Geometry: final body of the model. Coordinates: model frame, mm. Face numbers are marked on the shaded views. A direction names the side the tool comes from. Round coordinates to 2 decimals unless told otherwise and drop trailing zeros. Write each loop counter-clockwise with the first axis right and the second up, starting at its lowest first coordinate (ties: lowest second). Pieces come first, ordered by that corner, then holes. Notation, with made-up numbers: (79.25, 43.5) - (119.25, 43.5) arc R22 ccw to (119.25, 60.5) - close; hole circle Ø4 at (-5.5, 79.5). An arc over 180 degrees is marked (long way). Use a Markdown table: item, result. Add a question column.
```python
from build123d import *

# Parameters (mm, degrees)
SKETCH8_R           = 2
BOSS_EXTRUDE6_DEPTH = 9
BOSS_EXTRUDE7_START = -9
SKETCH9_R           = 1.395
BOSS_EXTRUDE7_DEPTH = 32
CHAMFER3_SIZE       = 3.5
BOSS_EXTRUDE8_START = -9
SKETCH11_R          = 2
BOSS_EXTRUDE8_DEPTH = 28.5
CUT_EXTRUDE1_START  = -0.2
CUT_EXTRUDE1_DEPTH  = 24.2
FILLET5_R           = 3.2


with BuildPart() as part:
    # Sketch8 → Boss-Extrude6 (new body, symmetric)
    with BuildSketch(Plane.XY):
        with BuildLine():
            Line((-16, -16.195281799), (-16, -22.05))
            Line((-16, -22.05), (16, -22.05))
            ThreePointArc((16, -22.05), (20.242640687, -20.292640687), (22, -16.05))
            Line((22, -16.05), (22, 16.05))
            Line((22, 16.05), (-1.424393869, 2.820825363))
            Line((-1.424393869, 2.820825363), (-1.424393869, -9.35))
            Line((-1.424393869, -9.35), (-1.949620424, -9.35))
            ThreePointArc((-1.949620424, -9.35), (-3.3, -11.095), (-4.650379576, -9.35))
            Line((-4.650379576, -9.35), (-16, -9.35))
            Line((-16, -9.35), (-16, -16.195281799))
        make_face()
        with Locations((16, -16.05)):
            Circle(SKETCH8_R, mode=Mode.SUBTRACT)
    extrude(amount=BOSS_EXTRUDE6_DEPTH, both=True)

    # Sketch9 → Boss-Extrude7 (add)
    with BuildSketch(Plane.XY.offset(BOSS_EXTRUDE7_START)):
        with BuildLine():
            Line((8.5, 4.678478311), (-5.487189769, -7.103420343))
            ThreePointArc((-5.487189769, -7.103420343), (-6.682635801, -9.410517634), (-5.896579657, -11.887189769))
            Line((-5.896579657, -11.887189769), (-0.72278451, -18.029396273))
            Line((-0.72278451, -18.029396273), (8.5, -12.820730998))
            Line((8.5, -12.820730998), (8.5, 4.678478311))
        make_face()
        with Locations((-3.3, -9.7)):
            Circle(SKETCH9_R, mode=Mode.SUBTRACT)
    extrude(amount=BOSS_EXTRUDE7_DEPTH)

    # Chamfer3
    chamfer3_edges = [part.edges().sort_by_distance(p)[0] for p in [
        (8.5, -4.071126344, 23),
    ]]
    chamfer(chamfer3_edges, length=CHAMFER3_SIZE)

    # Sketch11 → Boss-Extrude8 (add)
    with BuildSketch(Plane.XY.offset(BOSS_EXTRUDE8_START)):
        with BuildLine():
            Line((8.5, 8.425731957), (8.5, -22.05))
            Line((8.5, -22.05), (16, -22.05))
            ThreePointArc((16, -22.05), (20.242640687, -20.292640687), (22, -16.05))
            Line((22, -16.05), (22, 16.05))
            Line((22, 16.05), (8.5, 8.425731957))
        make_face()
        with Locations((16, -16.05)):
            Circle(SKETCH11_R, mode=Mode.SUBTRACT)
    extrude(amount=BOSS_EXTRUDE8_DEPTH)

    # Sketch8<4> → Cut-Extrude1 (cut, through all)
    with BuildSketch(Plane.XY.offset(CUT_EXTRUDE1_START)):
        Polygon((-16, -16.195281799), (-16, -22.05), (-14.391687016, -22.05), (-14.391687016, -9.35), (-16, -9.35), align=None)
    extrude(amount=CUT_EXTRUDE1_DEPTH, mode=Mode.SUBTRACT)

    # Fillet5
    fillet5_edges = [part.edges().sort_by_distance(p)[0] for p in [
        (-10.534298793, -9.35, 9),
        (-2.945843508, -22.05, 9),
    ]]
    fillet(fillet5_edges, radius=FILLET5_R)


solid = part.part
```
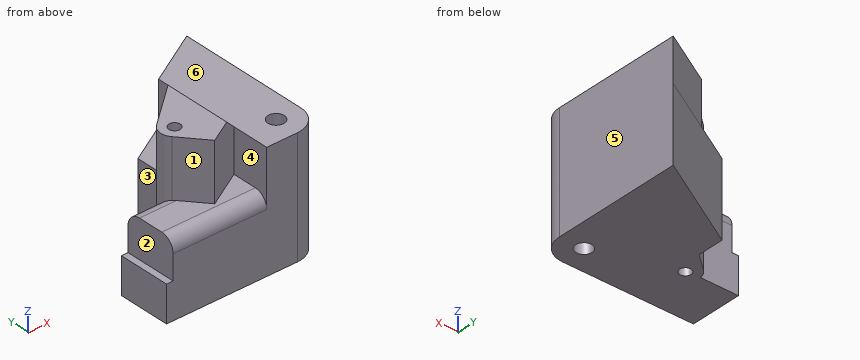
1) Section B-B, the plane z = 8. Return the cut outline in (x, y) (3 decimals), then the cut area to 3 significant figures.
2) Set-up query: the marked faces 1, 2 and 3. Return all of +Z, -Z, +X, -X, +Y, -Y with unobstructed straight access to the full face (end or side cutting, diameter ignored); none if empty.
3) Section D-D, the plane y = 0.5. Return the cut outline in (x, z), then the cut area to 3 significant figures.
4) Section C-C, the plane x = 3. Return the cut outline in (y, z).
5) Pin query (flat end, axial travel): P1, Ø0.8, axis at x = -15, y = -13.5, coming from the +Z side; P2, Ø10.5, axis at x = -12, z = 0.5, coming from the +Y side; P3, Ø1.5, axis at x = -6, z = 14, coming from the -Y side. Return the tip coordinate at first contact, or that it passes through.
6) Draft query along X for the marked faces 4, 5 and 6. Return one class per face: released by +X, released by -X, zero draft, split by the parting line, or undercut.
7) Section A-A, the plane y = -15.5. Return the cut outline in (x, z), then the cut area to 3 significant figures.
8) Material intervals for L1, parallel to X at y = -9.7, z = 8.5 (3 decimals); L2, parallel to X at y = -16, z = 13; L3, parallel to X at y = 2.5, z = 0.5, sorted ascending. Write a range as from..to.
Output values:
| question | item | result |
|---|---|---|
| 1 | outline | (-14.392, -21.174) - (8.5, -21.174) - (8.5, -22.05) - (16, -22.05) arc R6 ccw to (22, -16.05) - (22, 16.05) - (-1.424, 2.821) - (-1.424, -3.681) - (-5.487, -7.103) arc R3.395 ccw to (-6.654, -10.226) - (-14.392, -10.226) - close; hole circle Ø2.79 at (-3.3, -9.7); hole circle Ø4 at (16, -16.05) |
| 1 | area | 867 mm^2 |
| 2 | face 1 | +Z, -X, -Y |
| 2 | face 2 | +Z, -X, +Y, -Y |
| 2 | face 3 | +Z, -Z, -X, +Y |
| 3 | outline | (-1.42, -9) - (22, -9) - (22, 19.5) - (8.5, 19.5) - (5, 23) - (3.54, 23) - (3.54, 9) - (-1.42, 9) - close |
| 3 | area | 627 mm^2 |
| 4 | outline | (-22.05, -9) - (5.32, -9) - (5.32, 9) - (0.05, 9) - (0.05, 23) - (-15.93, 23) - (-15.93, 9) - (-18.85, 9) arc R3.2 ccw to (-22.05, 5.8) - close |
| 5 | P1 | stops at z = -0.2 |
| 5 | P2 | stops at y = -9.35 |
| 5 | P3 | stops at y = -12.65 |
| 6 | face 4 | undercut |
| 6 | face 5 | released by +X |
| 6 | face 6 | zero draft |
| 7 | outline | (-16, -9) - (14.08, -9) - (14.08, 19.5) - (8.5, 19.5) - (8.5, 9) - (3.76, 9) - (3.76, 23) - (-2.85, 23) - (-2.85, 9) - (-14.39, 9) - (-14.39, -0.2) - (-16, -0.2) - close; (17.92, -9) - (22, -9) - (22, 19.5) - (17.92, 19.5) - close |
| 7 | area | 794 mm^2 |
| 8 | L1 | x = -6.695..-4.695, -1.905..22 |
| 8 | L2 | x = -2.43..2.87, 8.5..14, 18..22 |
| 8 | L3 | x = -1.42..22 |
